from build123d import *

# Parameters (mm, degrees)
BOSS_EXTRUDE1_DEPTH        = 3.175
SKETCH2_R                  = 2.5
CUT_EXTRUDE2_DEPTH         = 10
SKETCH8_W                  = 3.175
SKETCH8_H                  = 3.175
BOSS_EXTRUDE2_DEPTH        = 80
CONVERT_SOLID2_START       = 2.233560192
CONVERT_SOLID2_OUTLINE_W   = 3.175
CONVERT_SOLID2_OUTLINE_H   = 23.379999999
CONVERT_SOLID2_OUTLINE_H_2 = 19.120000001
CONVERT_SOLID2_OUTLINE_H_3 = 15
CONVERT_SOLID2_DEPTH       = 0.941439808
CONVERT_SOLID2_START_2     = -3.2
CONVERT_SOLID2_2_OUTLINE_R = 2.5
CONVERT_SOLID2_2_DEPTH     = 3.650867885
CONVERT_SOLID2_START_3     = -80
CONVERT_SOLID2_3_OUTLINE_W = 0.025
CONVERT_SOLID2_3_OUTLINE_H = 80
CONVERT_SOLID2_3_DEPTH     = 77.404032
CONVERT_SOLID2_START_4     = 3.175
CONVERT_SOLID2_4_OUTLINE_R = 2.5
CONVERT_SOLID2_4_DEPTH     = 0.025
CONVERT_SOLID2_START_5     = -54.620000001
CONVERT_SOLID2_5_DEPTH     = 67.5
CONVERT_SOLID2_START_6     = -67.120000001
CONVERT_SOLID2_6_DEPTH     = 80
CONVERT_SOLID2_START_7     = 24.325
CONVERT_SOLID2_7_OUTLINE_R = 2.5
CONVERT_SOLID2_7_DEPTH     = 0.675
FILLET1_R                  = 10


with BuildPart() as part:
    # Sketch1 → Boss-Extrude1 (new body)
    with BuildSketch(Plane.XY):
        Polygon((-58.85, 12.879999999), (-58.85, -27.120000001), (1.15, -67.120000001), (21.15, -67.120000001), (21.15, 12.879999999), align=None)
    extrude(amount=BOSS_EXTRUDE1_DEPTH)

    # Sketch2 → Cut-Extrude2 (cut)
    with BuildSketch(Plane.XY.offset(3.175)):
        with Locations((-48.85, 2.879999999)):
            Circle(SKETCH2_R)
        with Locations((-48.85, -17.12)):
            Circle(SKETCH2_R)
        with Locations((-28.85, 2.879999999)):
            Circle(SKETCH2_R)
        with BuildLine():
            Line((8.65, -54.620000001), (13.65, -54.620000001))
            ThreePointArc((13.65, -54.620000001), (16.15, -57.120000001), (13.65, -59.620000001))
            Line((13.65, -59.620000001), (8.65, -59.620000001))
            ThreePointArc((8.65, -59.620000001), (6.15, -57.120000001), (8.65, -54.620000001))
        make_face()
        with BuildLine():
            Line((8.65, -34.620000001), (13.65, -34.620000001))
            ThreePointArc((13.65, -34.620000001), (16.15, -37.120000001), (13.65, -39.620000001))
            Line((13.65, -39.620000001), (8.65, -39.620000001))
            ThreePointArc((8.65, -39.620000001), (6.15, -37.120000001), (8.65, -34.620000001))
        make_face()
        with BuildLine():
            Line((-5.5, -15.5), (-9.5, -15.5))
            ThreePointArc((-9.5, -15.5), (-12, -13), (-9.5, -10.5))
            Line((-9.5, -10.5), (-5.5, -10.5))
            ThreePointArc((-5.5, -10.5), (-3, -13), (-5.5, -15.5))
        make_face()
        with BuildLine():
            Line((0.5, -10.5), (4.5, -10.5))
            ThreePointArc((4.5, -10.5), (7, -13), (4.5, -15.5))
            Line((4.5, -15.5), (0.5, -15.5))
            ThreePointArc((0.5, -15.5), (-2, -13), (0.5, -10.5))
        make_face()
    extrude(amount=-CUT_EXTRUDE2_DEPTH, mode=Mode.SUBTRACT)


with BuildPart() as body_2:
    # Mirror1: mirrored copy
    add(part.part.mirror(Plane(origin=(10.575, 0, -10.575), x_dir=(0.7071067811865489, 0, 0.7071067811865462), z_dir=(0.7071067811865464, 0, -0.7071067811865488))))


with BuildPart() as part_1:
    add(part.part)

    add(body_2.part)  # Boss-Extrude2 merges body 2
    # Sketch8 → Boss-Extrude2 (add, through all)
    with BuildSketch(Plane(origin=(0, 12.879999999, 0), x_dir=(1, 0, 0), z_dir=(0, 1, 0))):
        with Locations((22.7375, -1.5875)):
            Rectangle(SKETCH8_W, SKETCH8_H)
    extrude(amount=-BOSS_EXTRUDE2_DEPTH)

    # Convert-Solid2: read off the stored shape, not the designer's step
    # Convert-Solid2 outline → Convert-Solid2 (cut)
    with BuildSketch(Plane.XY.offset(CONVERT_SOLID2_START)):
        with Locations((22.7375, 1.19)):
            Rectangle(CONVERT_SOLID2_OUTLINE_W, CONVERT_SOLID2_OUTLINE_H)
        with Locations((22.7375, -25.060000001)):
            Rectangle(CONVERT_SOLID2_OUTLINE_W, CONVERT_SOLID2_OUTLINE_H_2)
        with Locations((22.7375, -47.120000001)):
            Rectangle(CONVERT_SOLID2_OUTLINE_W, CONVERT_SOLID2_OUTLINE_H_3)
    extrude(amount=CONVERT_SOLID2_DEPTH, mode=Mode.SUBTRACT)

    # Convert-Solid2 2 outline → Convert-Solid2 2 (add)
    with BuildSketch(Plane.XY.offset(CONVERT_SOLID2_START_2)):
        Polygon((21.15, 12.879999999), (-58.85, 12.879999999), (-58.85, -27.120000001), (1.15, -67.120000001), (21.15, -67.120000001), align=None)
        with BuildLine():
            Line((13.65, -59.620000001), (8.65, -59.620000001))
            ThreePointArc((8.65, -59.620000001), (6.15, -57.120000001), (8.65, -54.620000001))
            Line((8.65, -54.620000001), (13.65, -54.620000001))
            ThreePointArc((13.65, -54.620000001), (16.15, -57.120000001), (13.65, -59.620000001))
        make_face(mode=Mode.SUBTRACT)
        with BuildLine():
            Line((13.65, -39.620000001), (8.65, -39.620000001))
            ThreePointArc((8.65, -39.620000001), (6.15, -37.120000001), (8.65, -34.620000001))
            Line((8.65, -34.620000001), (13.65, -34.620000001))
            ThreePointArc((13.65, -34.620000001), (16.15, -37.120000001), (13.65, -39.620000001))
        make_face(mode=Mode.SUBTRACT)
        with Locations((-48.85, -17.12)):
            Circle(CONVERT_SOLID2_2_OUTLINE_R, mode=Mode.SUBTRACT)
        with Locations((-48.85, 2.879999999)):
            Circle(CONVERT_SOLID2_2_OUTLINE_R, mode=Mode.SUBTRACT)
        with Locations((-28.85, 2.879999999)):
            Circle(CONVERT_SOLID2_2_OUTLINE_R, mode=Mode.SUBTRACT)
        with BuildLine():
            Line((-9.5, -10.5), (-5.5, -10.5))
            ThreePointArc((-5.5, -10.5), (-3, -13), (-5.5, -15.5))
            Line((-5.5, -15.5), (-9.5, -15.5))
            ThreePointArc((-9.5, -15.5), (-12, -13), (-9.5, -10.5))
        make_face(mode=Mode.SUBTRACT)
        with BuildLine():
            Line((0.5, -10.5), (4.5, -10.5))
            ThreePointArc((4.5, -10.5), (7, -13), (4.5, -15.5))
            Line((4.5, -15.5), (0.5, -15.5))
            ThreePointArc((0.5, -15.5), (-2, -13), (0.5, -10.5))
        make_face(mode=Mode.SUBTRACT)
    extrude(amount=CONVERT_SOLID2_2_DEPTH)

    # Convert-Solid2 3 outline → Convert-Solid2 3 (add)
    with BuildSketch(Plane.XY.offset(CONVERT_SOLID2_START_3)):
        with Locations((24.3375, -27.120000001)):
            Rectangle(CONVERT_SOLID2_3_OUTLINE_W, CONVERT_SOLID2_3_OUTLINE_H)
    extrude(amount=CONVERT_SOLID2_3_DEPTH)

    # Convert-Solid2 4 outline → Convert-Solid2 4 (add)
    with BuildSketch(Plane.XY.offset(CONVERT_SOLID2_START_4)):
        Polygon((21.15, 12.879999999), (-58.85, 12.879999999), (-58.85, -27.120000001), (1.15, -67.120000001), (21.15, -67.120000001), align=None)
        with BuildLine():
            Line((13.65, -59.620000001), (8.65, -59.620000001))
            ThreePointArc((8.65, -59.620000001), (6.15, -57.120000001), (8.65, -54.620000001))
            Line((8.65, -54.620000001), (13.65, -54.620000001))
            ThreePointArc((13.65, -54.620000001), (16.15, -57.120000001), (13.65, -59.620000001))
        make_face(mode=Mode.SUBTRACT)
        with BuildLine():
            Line((13.65, -39.620000001), (8.65, -39.620000001))
            ThreePointArc((8.65, -39.620000001), (6.15, -37.120000001), (8.65, -34.620000001))
            Line((8.65, -34.620000001), (13.65, -34.620000001))
            ThreePointArc((13.65, -34.620000001), (16.15, -37.120000001), (13.65, -39.620000001))
        make_face(mode=Mode.SUBTRACT)
        with Locations((-48.85, -17.12)):
            Circle(CONVERT_SOLID2_4_OUTLINE_R, mode=Mode.SUBTRACT)
        with Locations((-48.85, 2.879999999)):
            Circle(CONVERT_SOLID2_4_OUTLINE_R, mode=Mode.SUBTRACT)
        with Locations((-28.85, 2.879999999)):
            Circle(CONVERT_SOLID2_4_OUTLINE_R, mode=Mode.SUBTRACT)
        with BuildLine():
            Line((-9.5, -10.5), (-5.5, -10.5))
            ThreePointArc((-5.5, -10.5), (-3, -13), (-5.5, -15.5))
            Line((-5.5, -15.5), (-9.5, -15.5))
            ThreePointArc((-9.5, -15.5), (-12, -13), (-9.5, -10.5))
        make_face(mode=Mode.SUBTRACT)
        with BuildLine():
            Line((0.5, -10.5), (4.5, -10.5))
            ThreePointArc((4.5, -10.5), (7, -13), (4.5, -15.5))
            Line((4.5, -15.5), (0.5, -15.5))
            ThreePointArc((0.5, -15.5), (-2, -13), (0.5, -10.5))
        make_face(mode=Mode.SUBTRACT)
    extrude(amount=CONVERT_SOLID2_4_DEPTH)

    # Convert-Solid2 5 outline → Convert-Solid2 5 (add)
    with BuildSketch(Plane(origin=(0, 0, 0), x_dir=(1, 0, 0), z_dir=(0, 1, 0)).offset(CONVERT_SOLID2_START_5)):
        with BuildLine():
            Line((21.15, -2.233560192), (21.15, -2.342562585))
            ThreePointArc((21.15, -2.342562585), (21.241340362, -2.288813955), (21.331778178, -2.233560192))
            Line((21.331778178, -2.233560192), (21.15, -2.233560192))
        make_face()
    extrude(amount=CONVERT_SOLID2_5_DEPTH)

    # Convert-Solid2 6 outline → Convert-Solid2 6 (cut)
    with BuildSketch(Plane(origin=(0, 0, 0), x_dir=(1, 0, 0), z_dir=(0, 1, 0)).offset(CONVERT_SOLID2_START_6)):
        with BuildLine():
            Line((-58.85, 3.2), (-58.85, 0))
            Line((-58.85, 0), (17.95, 0))
            ThreePointArc((17.95, 0), (20.2127417, 0.9372583), (21.15, 3.2))
            Line((21.15, 3.2), (-58.85, 3.2))
        make_face()
        with BuildLine():
            Line((17.95, -3.2), (21.15, -3.2))
            Line((21.15, -3.2), (21.15, -3.175))
            Line((21.15, -3.175), (24.325, -3.175))
            Line((24.325, -3.175), (24.325, 2.595968))
            Line((24.325, 2.595968), (24.35, 2.595968))
            Line((24.35, 2.595968), (24.35, 3.2))
            ThreePointArc((24.35, 3.2), (22.4754834, -1.3254834), (17.95, -3.2))
        make_face()
    extrude(amount=CONVERT_SOLID2_6_DEPTH, mode=Mode.SUBTRACT)

    # Convert-Solid2 7 outline → Convert-Solid2 7 (cut)
    with BuildSketch(Plane.YZ.offset(CONVERT_SOLID2_START_7)):
        Polygon((-27.120000001, -80), (-67.120000001, -20), (-67.120000001, -80), align=None)
        with BuildLine():
            Line((-59.620000001, -7.5), (-59.620000001, -12.5))
            ThreePointArc((-59.620000001, -12.5), (-57.120000001, -15), (-54.620000001, -12.5))
            Line((-54.620000001, -12.5), (-54.620000001, -7.5))
            ThreePointArc((-54.620000001, -7.5), (-57.120000001, -5), (-59.620000001, -7.5))
        make_face()
        with BuildLine():
            Line((-39.620000001, -7.5), (-39.620000001, -12.5))
            ThreePointArc((-39.620000001, -12.5), (-37.120000001, -15), (-34.620000001, -12.5))
            Line((-34.620000001, -12.5), (-34.620000001, -7.5))
            ThreePointArc((-34.620000001, -7.5), (-37.120000001, -5), (-39.620000001, -7.5))
        make_face()
        with BuildLine():
            Line((-10.5, -30.65), (-10.5, -26.65))
            ThreePointArc((-10.5, -26.65), (-13, -24.15), (-15.5, -26.65))
            Line((-15.5, -26.65), (-15.5, -30.65))
            ThreePointArc((-15.5, -30.65), (-13, -33.15), (-10.5, -30.65))
        make_face()
        with BuildLine():
            Line((-10.5, -20.65), (-10.5, -16.65))
            ThreePointArc((-10.5, -16.65), (-13, -14.15), (-15.5, -16.65))
            Line((-15.5, -16.65), (-15.5, -20.65))
            ThreePointArc((-15.5, -20.65), (-13, -23.15), (-10.5, -20.65))
        make_face()
        with Locations((2.879999999, -50)):
            Circle(CONVERT_SOLID2_7_OUTLINE_R)
        with Locations((-17.12, -70)):
            Circle(CONVERT_SOLID2_7_OUTLINE_R)
        with Locations((2.879999999, -70)):
            Circle(CONVERT_SOLID2_7_OUTLINE_R)
    extrude(amount=CONVERT_SOLID2_7_DEPTH, mode=Mode.SUBTRACT)

    # Fillet1
    fillet1_edges = [part_1.edges().sort_by_distance(p)[0] for p in [
        (1.15, -67.120000001, 1.5875),
        (22.7375, -67.120000001, -20),
        (22.7375, -27.120000001, -80),
        (22.7375, 12.879999999, -80),
        (-58.85, 12.879999999, 1.5875),
        (-58.85, -27.120000001, 1.5875),
    ]]
    fillet(fillet1_edges, radius=FILLET1_R)


solid = part_1.part
CAD build for the part. Positions are in the model's coordinates, mm. A direction names the side the tool comes from. Coordinates: 2 decimals unless noted, no trailing zeros. Order: outer loops, then holes, each group sorted by start corner. A loop starts at its lowest first (then second) coordinate and runs counter-clockwise, first axis right, second up. Notation, with made-up numbers: (69.25, -21) -> (120.25, -21) arc R29 ccw to (120.25, 15) -> close; hole circle Ø1 at (-29, -33.5). An arc over 180 degrees is marked (long way). Answer in a Markdown table with one row per item.
1) Band-saw the part on A-A (y = -57.12). List the corners of the cut face in (x, z), and give its area (3 significant figures).
Check values:
| item | result |
|---|---|
| outline | (-13.85, 0) -> (6.15, 0) -> (6.15, 3.2) -> (-13.85, 3.2) -> close; (16.15, 0) -> (17.95, 0) arc R3.2 cw to (21.15, -3.2) -> (21.15, -5) -> (24.35, -5) -> (24.35, -3.2) arc R6.4 ccw to (17.95, 3.2) -> (16.15, 3.2) -> close; (21.15, -35) -> (24.35, -35) -> (24.35, -15) -> (21.15, -15) -> close |
| area | 164 mm2 |
2) Which spindle directions (+Z, -Z, +X, -X, +Y, -Y) get a long thin tool onto all of the face, cutting with end or side? Do faces 1 (the face through (23, -59.62, -10)), 2 (the face through (-57.699, -26.426, 1.622)), 3 (the face through (6.15, -37.17, 1.58)). Say none if no direction does.
Check values:
| item | result |
|---|---|
| face 1 | +X, -X |
| face 2 | +Z, -Z, -X, -Y |
| face 3 | +Z, -Z |
3) Mould opens along Z. For faces 4 (the face through (23, -15.5, -29)), 5 (the face through (22.772, -26.547, -78.784)), 6 (the face through (-56, 9.87, 1.62)) say: pulls with the +Z half, pulls with the -Z half, needs draft (parallel to the pull), parting line crosses it, or undercut.
Check values:
| item | result |
|---|---|
| face 4 | undercut |
| face 5 | pulls with the -Z half |
| face 6 | needs draft |
4) Band-saw the part on D-D (z = -58.5). List the corners of the cut face in (x, y), and give its area (3 significant figures).
Check values:
| item | result |
|---|---|
| outline | (21.15, -41.45) -> (24.35, -41.45) -> (24.35, 12.88) -> (21.15, 12.88) -> close |
| area | 174 mm2 |
5) Band-saw the part on B-B (y = -17.12). List the corners of the cut face in (x, z).
Check values:
| item | result |
|---|---|
| outline | (-58.85, 0) -> (-51.35, 0) -> (-51.35, 3.2) -> (-58.85, 3.2) -> close; (-46.35, 0) -> (17.95, 0) arc R3.2 cw to (21.15, -3.2) -> (21.15, -67.5) -> (24.35, -67.5) -> (24.35, -3.2) arc R6.4 ccw to (21.33, 2.23) arc R6.4 ccw to (21.15, 2.34) arc R6.4 ccw to (17.95, 3.2) -> (-46.35, 3.2) -> close; (21.15, -80) -> (24.35, -80) -> (24.35, -72.5) -> (21.15, -72.5) -> close |
6) Drill centre lines: line 1 (Y direction, x = -48, z = 2); line 2 (Z direction, x = 23.1, y = 2.88); line 3 (Y direction, x = -48.85, z = 2.1). Where is each one in solid material? Low to high.
Check values:
| item | result |
|---|---|
| line 1 | -34.35 to -19.47, -14.77 to 0.53, 5.23 to 12.88 |
| line 2 | -80 to -72.5, -67.5 to -52.5, -47.5 to 0.6 |
| line 3 | -33.79 to -19.62, -14.62 to 0.38, 5.38 to 12.88 |
7) Band-saw the part on C-C (x = -17). List the corners of the cut face in (y, z), and give its area (3 significant figures).
Check values:
| item | result |
|---|---|
| outline | (-55.02, 0) -> (12.88, 0) -> (12.88, 3.2) -> (-55.02, 3.2) -> close |
| area | 217 mm2 |
8) Flat gauge pins, fed straight in: P1, Ø8, axis at x = -48.85, y = -17.12, coming from the -Z side; P2, Ø6, axis at y = 5, z = -11.5, coming from the -X side; P3, Ø3, axis at x = -28.85, y = 2.88, coming from the +Z side; P4, Ø1, axis at x = 22.5, z = -28, coming from the -Y side. Where does each tip first touch, or does it go through?
Check values:
| item | result |
|---|---|
| P1 | z = 0 |
| P2 | x = 21.15 |
| P3 | through |
| P4 | y = -62.12 |
